```python
from build123d import *

# Parameters (mm, degrees)
SKETCH2_R           = 1.5
BOSS_EXTRUDE1_DEPTH = 6
CHAMFER1_SIZE       = 0.3
CUT_EXTRUDE1_DEPTH  = 1.2
SKETCH8_R           = 1.204700538
CUT_EXTRUDE2_DEPTH  = 1
CUT_EXTRUDE2_TAPER  = 45


with BuildPart() as part:
    # Sketch2 → Boss-Extrude1 (new body)
    with BuildSketch(Plane(origin=(0, 0, 0), x_dir=(0, 0, -1), z_dir=(1, 0, 0))):
        Circle(SKETCH2_R)
    extrude(amount=-BOSS_EXTRUDE1_DEPTH)

    # Chamfer1
    chamfer1_edges = [part.edges().sort_by_distance(p)[0] for p in [
        (0, 0, 1.5),
    ]]
    chamfer(chamfer1_edges, length=CHAMFER1_SIZE)

    # Sketch6 → Revolve1 (revolve)
    with BuildSketch(Plane.XY):
        with BuildLine():
            Line((-7.65, 0), (-7.65, 1.5))
            ThreePointArc((-7.65, 1.5), (-7.055944823, 2.284868705), (-6.25, 2.85))
            Line((-6.25, 2.85), (-6, 2.85))
            Line((-6, 2.85), (-6, 0))
            Line((-6, 0), (-7.65, 0))
        make_face()
    revolve(axis=Axis((-6, 0, 0), (-1, 0, 0)))

    # Sketch7 → Cut-Extrude1 (cut)
    with BuildSketch(Plane.ZY.offset(7.65)):
        Polygon((0, 1.154700538), (-1, 0.577350269), (-1, -0.577350269), (0, -1.154700538), (1, -0.577350269), (1, 0.577350269), align=None)
    extrude(amount=-CUT_EXTRUDE1_DEPTH, mode=Mode.SUBTRACT)

    # Sketch8 → Cut-Extrude2 (cut)
    with BuildSketch(Plane.ZY.offset(7.65)):
        Circle(SKETCH8_R)
    extrude(amount=-CUT_EXTRUDE2_DEPTH, taper=CUT_EXTRUDE2_TAPER, mode=Mode.SUBTRACT)


solid = part.part
```
Source: CAD feature listing. Evaluate the final solid. Frame: model axes, mm. A direction names the side the tool comes from. Coordinates: 2 decimals unless noted, no trailing zeros. Loops run counter-clockwise (first coordinate to the right, second up) from the corner with the lowest first, then second, coordinate; pieces in that order, holes last. Notation, with made-up numbers: (36.5, 2.25) - (43.5, 2.25) arc R18 ccw to (43.5, 28.25) - close; hole circle Ø5 at (4, 33). An arc over 180 degrees is marked (long way). Answer as CSV lines item,"result".
1. Mould query, pull axis Y, two halves, no side actions, for faces 3 (the cylindrical face through (-3.11, 0.07, 1.5)), 4 (the flat face through (-7.03, -0.87, 0.49)), 5 (the flat face through (-7.03, 0.86, 0.51)), 6 (the flat face through (0, 0, 0)). Classes: released by +Y, released by -Y, zero draft, split by the parting line, or undercut.
Established:
face 3,"split by the parting line"
face 4,"undercut"
face 5,"undercut"
face 6,"zero draft"
2. Reachability of faces 1 (the flat face through (-6, 1.2, 1.2)), 2 (the flat face through (-7, 0, -1)) from +Z, -Z, +X, -X, +Y, -Y: full face, straight path, thin tool, end or side. Return the list, or none.
Established:
face 1,"+X"
face 2,"-X"
3. Ray query, line 1 (Y direction, x = -4, z = 0.05); line 2 (Y direction, x = -7, z = -0.3); line 3 (Z direction, x = -7, y = -0.3). Return the intervals inside material, ascending.
Established:
line 1,"y = -1.5 to 1.5"
line 2,"y = -2.32 to -0.98, 0.98 to 2.32"
line 3,"z = -2.32 to -1, 1 to 2.32"
4. Section A-A (x = -4.75). Return loops of the section in (y, z), then the cut area to 3 significant figures.
Established:
outline,"circle Ø3 at (0, 0)"
area,"7.07 mm2"
5. Contact query for flat-ended pins moving along their axis: pin 1 (2 mm diameter, centred on x = -3, z = 0.5, fed in from -Y); pin 2 (0.6 mm diameter, centred on x = -7, y = 0, fed in from -Z); pin 3 (3 mm diameter, centred on x = -3, y = 1.5, fed in from -Z). Output: stop coordinate, or through.
Established:
pin 1,"stops at y = -1.5"
pin 2,"stops at z = -2.58"
pin 3,"stops at z = -1.5"
6. Section C-C (z = -2.3). Return loops of the section in (x, y), then the cut area to 3 significant figures.
Established:
outline,"(-6.25, -1.68) - (-6, -1.68) - (-6, 1.68) - (-6.25, 1.68) arc R2.19 ccw to start"
area,"2.69 mm2"
7. Section B-B (y = 2.2). Return loops of the section in (x, z).
Established:
outline,"(-6.25, -1.81) - (-6, -1.81) - (-6, 1.81) - (-6.25, 1.81) arc R2.29 ccw to start"
